```python
from build123d import *

# Parameters (mm, degrees)
F0_W     = 38.4
F0_H     = 129.5
F0_W_2   = 31.4
F0_H_2   = 111
F1_DEPTH = 2
F2_DEPTH = 35
F3_SIZE2 = 17.5
F3_SIZE  = 7.5
F4_SIZE2 = 32.99999
F4_SIZE  = 5.99999
F6_DEPTH = 35.001
F7_W     = 32.5
F7_H     = 12.5
F8_DEPTH = 1
F9_SIZE2 = 10
F9_SIZE  = 1


# Not quite as in the source:
# - a fillet or chamfer is up to 0.001 mm smaller than in the source, because OpenCascade refuses the exact size


with BuildPart() as f1:
    # F0 (on Top) → F1 (new body)
    with BuildSketch(Plane.XY):
        with Locations((0, -5.75)):
            Rectangle(F0_W, F0_H)
        Rectangle(F0_W_2, F0_H_2, mode=Mode.SUBTRACT)
        Rectangle(F0_W_2, F0_H_2)
    extrude(amount=F1_DEPTH)

    # F0 (on Top) → F2 (join)
    with BuildSketch(Plane.XY):
        with Locations((0, -5.75)):
            Rectangle(F0_W, F0_H)
        Rectangle(F0_W_2, F0_H_2, mode=Mode.SUBTRACT)
    extrude(amount=F2_DEPTH)

    # F3
    f3_edges = [f1.edges().sort_by_distance(p)[0] for p in [
        (0, -70.5, 35),
    ]]
    f3_side = f1.faces().sort_by_distance((0, -69.149266, 35))[0]
    chamfer(f3_edges, length=F3_SIZE, length2=F3_SIZE2, reference=f3_side)

    # F4 (size 6 and 33 in the source; OpenCascade refuses exactly that, so slightly less here)
    f4_edges = [f1.edges().sort_by_distance(p)[0] for p in [
        (0, -55.5, 35),
    ]]
    f4_side = f1.faces().sort_by_distance((17.920994, -2, 35))[0]
    chamfer(f4_edges, length=F4_SIZE, length2=F4_SIZE2, reference=f4_side)

    # F5 (on face) → F6 (cut, through all)
    with BuildSketch(Plane.XY.offset(35)):
        Polygon((19.2, -28.5), (19.2, 17), (16.95, 19.25), (16.95, -30.75), align=None)
    extrude(amount=-F6_DEPTH, mode=Mode.SUBTRACT)

    # F7 (on face) → F8 (cut)
    with BuildSketch(Plane(origin=(0, -65.8965517241, 28.2413793103), x_dir=(1, 0, 0), z_dir=(0, -0.91914503, 0.3939192986))):
        with Locations((0, -2.1665561422)):
            Rectangle(F7_W, F7_H)
    extrude(amount=-F8_DEPTH, mode=Mode.SUBTRACT)

    # F9
    f9_edges = [f1.edges().sort_by_distance(p)[0] for p in [
        (0, 55.5, 2),
    ]]
    f9_side = f1.faces().sort_by_distance((0, 0, 2))[0]
    chamfer(f9_edges, length=F9_SIZE, length2=F9_SIZE2, reference=f9_side)


solid = f1.part
```
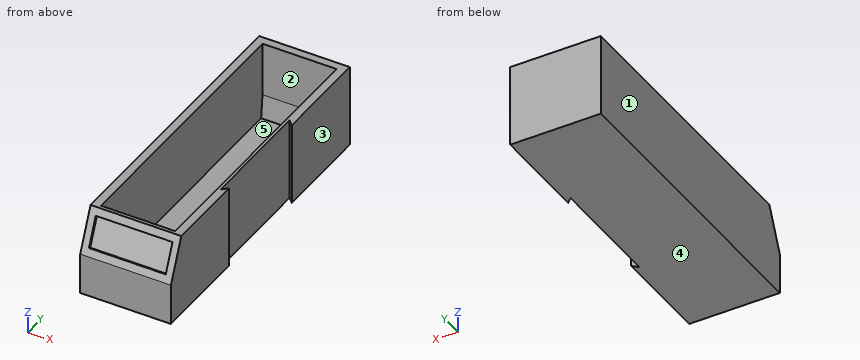
Can you work these out from the model? Positions are in its coordinate system, mm. Face numbers are marked on the shaded views. A direction names the side the tool comes from. Round coordinates to 2 decimals unless told otherwise and drop trailing zeros. Loops run counter-clockwise (first coordinate to the right, second up) from the corner with the lowest first, then second, coordinate; pieces in that order, holes last. Notation, with made-up numbers: M 79.5,-21 L 106.5,-21 A9 cw 106.5,-4 Z; hole C 32.5,77.25 d3. An arc over 180 degrees is marked long. Answer in a Markdown table with one row per item.
1. I'm going to push flat-ended pins straight in: pin 1 Ø5 at (y, z) = (-9.5, 27) entering from +X; pin 2 Ø11.5 at (x, z) = (3.5, 28) entering from -Y; pin 3 Ø4 at (x, z) = (-6, 27.5) entering from -Y. Where does each tip first touch, or does it pass through?
Established:
| item | result |
|---|---|
| pin 1 | x = 16.95 |
| pin 2 | y = -67.38 |
| pin 3 | y = -65.98 |
2. Please list where these lines run through material, in increasing order: line 1 (X direction, y = -40.5, z = 28); line 2 (X direction, y = -25, z = 13); line 3 (X direction, y = 19, z = 23). Write a range as from..to.
Established:
| item | result |
|---|---|
| line 1 | -19.2..-15.7, 15.7..19.2 |
| line 2 | -19.2..-15.7, 15.7..16.95 |
| line 3 | -19.2..-15.7, 15.7..16.95, 17.2..19.2 |
3. If we section it at D-D, the plane y = -4: Please give me the cut outline in (x, z), plus the area to 3 significant figures.
Established:
| item | result |
|---|---|
| outline | M -19.2,0 L 16.95,0 L 16.95,35 L 15.7,35 L 15.7,2 L -15.7,2 L -15.7,35 L -19.2,35 Z |
| area | 229 mm² |
4. If we section it at A-A, the plane y = -37: Please give me the cut outline in (x, z).
Established:
| item | result |
|---|---|
| outline | M -19.2,0 L 19.2,0 L 19.2,35 L 15.7,35 L 15.7,2 L -15.7,2 L -15.7,35 L -19.2,35 Z |
5. Thinking about a two-plate mould opening in X: for the marked faces 3, 4 and 5, which applies, pulls with the +X half, pulls with the -X half, needs draft (parallel to the pull), parting line crosses it, or undercut?
Established:
| item | result |
|---|---|
| face 3 | pulls with the +X half |
| face 4 | needs draft |
| face 5 | undercut |
6. On a 3-axis mill with a long thin cutter (end or side, diameter ignored), from which of +Z, -Z, +X, -X, +Y, -Y can I reach the whole of each face in a straight line? I mean the marked faces 1 and 2. Say none if no direction works.
Established:
| item | result |
|---|---|
| face 1 | +Z, -Z, -X, +Y, -Y |
| face 2 | +Z |
7. If we section it at B-B, the plane z = 22: Please give me the cut outline in (x, y).
Established:
| item | result |
|---|---|
| outline | M -19.2,-68.57 L -16.25,-68.57 L -16.25,-67.48 L 16.25,-67.48 L 16.25,-68.57 L 19.2,-68.57 L 19.2,-28.5 L 16.95,-30.75 L 16.95,19.25 L 19.2,17 L 19.2,59 L -19.2,59 Z; hole M -15.7,-59.14 L 15.7,-59.14 L 15.7,55.5 L -15.7,55.5 Z |
